Part model, mm, in its own coordinate system. Face numbers are marked on the shaded views. A direction names the side the tool comes from. Give positions to 0.01 mm unless a question says otherwise; leave off trailing zeros. Order: outer loops, then holes, each group sorted by start corner. A loop starts at its lowest first (then second) coordinate and runs counter-clockwise, first axis right, second up. Notation, with made-up numbers: M 23.5,25 L 53.5,25 A11 ccw 53.5,43 Z; hole C -2.5,86.25 d6. An arc over 180 degrees is marked long. Return JSON: item names as keys, results as strings.
Autodesk Inventor part; units mm, degrees
ref_plane "YZ Plane" through (0, 0, 0) normal (1, 0, 0) x (0, 1, 0)
ref_plane "XZ Plane" through (0, 0, 0) normal (0, 1, 0) x (-1, 0, 0)
ref_plane "XY Plane" through (0, 0, 0) normal (0, 0, 1) x (1, 0, 0)
sketch "Sketch1" plane through (0, 0, 0) normal (0, 0, 1) x (1, 0, 0)
  arc A0 (1.651, 0) -> (-1.651, 0) centre (0, 0) ccw
  arc A1 (1.651, 41.91) -> (-1.651, 41.91) centre (0, 41.91) ccw
  arc A2 (1.143, 45.4111) -> (-1.651, 38.6178) centre (0, 41.91) ccw
  line L0 (3.683, 48.26) -> (27.4676, 48.26)
  line L1 (27.4676, 6.35) -> (3.683, 6.35)
  line L2 (3.683, 6.35) -> (3.683, 48.26)
  line L3 (3.4296, 3.175) -> (3.4296, 0)
  line L4 (1.651, 38.904) -> (1.651, 3.2922)
  line L5 (1.143, 45.4111) -> (1.143, 50.292)
  line L6 (1.143, 50.292) -> (29.4996, 50.292)
  line L7 (29.4996, 50.292) -> (29.4996, 43.18)
  line L8 (29.4996, 43.18) -> (27.4676, 43.18)
  line L9 (3.4296, 3.175) -> (29.4996, 3.175)
  line L10 (29.4996, 3.175) -> (29.4996, 10.16)
  line L11 (29.4996, 10.16) -> (27.4676, 10.16)
  line L12 (27.4676, 48.26) -> (27.4676, 43.18)
  line L13 (27.4676, 10.16) -> (27.4676, 6.35)
  line L14 (1.651, 38.904) -> (1.651, 41.91)
  line L15 (-1.651, 41.91) -> (-1.651, 38.6178)
  line L16 (-1.651, 0) -> (-1.651, -3.2922)
  line L17 (1.651, 0) -> (1.651, -3.006)
  arc A3 (1.651, 3.2922) -> (-1.651, -3.2922) centre (0, 0) ccw
  arc A4 (1.651, -3.006) -> (3.4296, 0) centre (0, 0) ccw
  dimension "d0" = 3.302
  dimension "d2" = 41.91
  dimension "d4" = 6.35
  dimension "d5" = 6.35
  dimension "d6" = 3.683
  dimension "d7" = 2.54
  dimension "d8" = 2.032
  dimension "d9" = 2.032
  dimension "d10" = 5.08
  dimension "d11" = 3.81
  dimension "d12" = 3.175
  dimension "d13" = 2.032
extrude "Extrusion1" add sketch "Sketch1" along normal blind 3.81
fillet "Fillet1" radius 0.635 4 edges at (3.683, 48.26, 1.905) (3.683, 6.35, 1.905) (27.4676, 6.35, 1.905) (27.4676, 48.26, 1.905)
fillet "Fillet2" radius 1.905 6 edges at (1.143, 45.4111, 1.905) (1.651, 3.2922, 1.905) (3.4296, 3.175, 1.905) (29.4996, 50.292, 1.905) (1.143, 50.292, 1.905) (29.4996, 3.175, 1.905)
fillet "Fillet3" radius 0.508 3 edges at (1.651, -3.006, 1.905) (-1.651, -3.2922, 1.905) (-1.651, 38.6178, 1.905)
fillet "Fillet4" radius 0.508 4 edges at (27.4676, 10.16, 1.905) (27.4676, 43.18, 1.905) (29.4996, 43.18, 1.905) (29.4996, 10.16, 1.905)
properties part number "batteryHolderBracket" material "ABS Plastic"
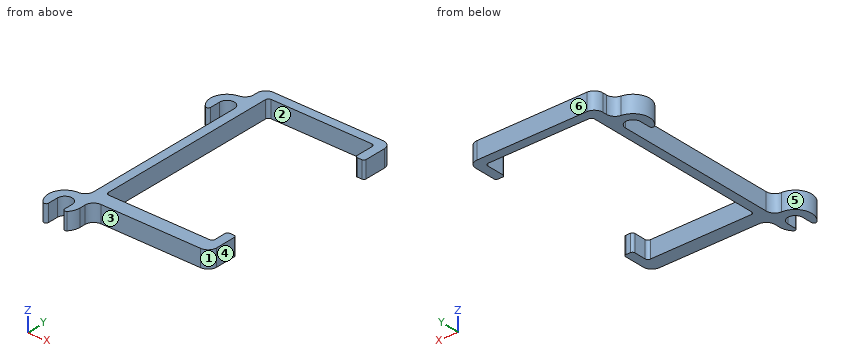
Q1. Band-saw the part on A-A (x = 18). Give the cut face in (y, z) (3 decimals).
Established:
{"outline": "M 3.175,0 L 6.35,0 L 6.35,3.81 L 3.175,3.81 Z; M 48.26,0 L 50.292,0 L 50.292,3.81 L 48.26,3.81 Z"}
Q2. 3-axis set-ups, long thin cutter, end or side, ignore diameter. For the marked faces 1 and 2: which of +Z, -Z, +X, -X, +Y, -Y reach the whole face in a straight line?
Established:
{"face 1": "+Z, -Z, +X, -Y", "face 2": "+Z, -Z"}
Q3. Band-saw the part on C-C (y = 22). Give the cut face in (x, z), then the cut area to 3 significant figures.
Established:
{"outline": "M 1.65,0 L 3.68,0 L 3.68,3.81 L 1.65,3.81 Z", "area": "7.74 mm²"}
Q4. Probe line 1 along Y through (x, z) = (25, 1.45) (3 decimals); line 2 along X through (y, z) = (0, 2.2); line 3 along X through (y, z) = (36.5, 2.2). List the from-to ranges inside material, lowest first.
Established:
{"line 1": "y = 3.175 to 6.35, 48.26 to 50.292", "line 2": "x = -3.68 to -1.65, 1.65 to 3.43", "line 3": "x = 1.65 to 3.68"}
Q5. Pin check, flat tips, straight feed: pin 1 (0.5 mm diameter, centred on x = 28.5, z = 2, fed in from +Y); pin 2 (2 mm diameter, centred on y = 41, z = 1.5, fed in from +X); pin 3 (0.7 mm diameter, centred on y = -0.5, z = 1, fed in from +X). Stop position of each tip, or through.
Established:
{"pin 1": "stops at y = 50.18", "pin 2": "stops at x = 3.68", "pin 3": "stops at x = 3.43"}
Q6. Band-saw the part on B-B (y = 9). Give the cut face in (x, z).
Established:
{"outline": "M 1.65,0 L 3.68,0 L 3.68,3.81 L 1.65,3.81 Z; M 27.47,0 L 29.5,0 L 29.5,3.81 L 27.47,3.81 Z"}
Q7. Two-plate mould, pull along Y, no slides. Class the marked faces 3, 4, 5 and 6: +Y half, -Y half, draft (parallel to the pull), parting line (faces both ways), or undercut.
Established:
{"face 3": "-Y half", "face 4": "draft", "face 5": "undercut", "face 6": "+Y half"}
